Source: CAD feature listing. Evaluate the final solid. Frame: model axes, mm. A direction names the side the tool comes from. Give positions to 0.01 mm unless a question says otherwise; leave off trailing zeros. Order: outer loops, then holes, each group sorted by start corner. A loop starts at its lowest first (then second) coordinate and runs counter-clockwise, first axis right, second up. Notation, with made-up numbers: (-4.75, 19) -> (43.25, 19) arc R19 cw to (43.25, 38) -> close; hole circle Ø6 at (26, 9.5). An arc over 180 degrees is marked (long way). Use CSV: the item, a comma, the result in double quotes.
```python
from build123d import *

# Parameters (mm, degrees)
SKETCH1_R                = 7.6
BOSS_EXTRUDE1_DEPTH      = 2
M4_CLEARANCE_HOLE1_D     = 4.3
M4_CLEARANCE_HOLE1_DEPTH = 8
M4_CLEARANCE_HOLE1_TIP   = 1.291850331


with BuildPart() as part:
    # Sketch1 → Boss-Extrude1 (new body)
    with BuildSketch(Plane(origin=(0, 0, 0), x_dir=(1, 0, 0), z_dir=(0, 1, 0))):
        with BuildLine():
            ThreePointArc((-4.926264158, -18.505524079), (0, -22.65), (4.926264158, -18.505524079))
            ThreePointArc((4.926264158, -18.505524079), (13.54109486, -13.54109486), (18.505524079, -4.926264158))
            ThreePointArc((18.505524079, -4.926264158), (22.65, 0), (18.505524079, 4.926264158))
            ThreePointArc((18.505524079, 4.926264158), (13.54109486, 13.54109486), (4.926264158, 18.505524079))
            ThreePointArc((4.926264158, 18.505524079), (0, 22.65), (-4.926264158, 18.505524079))
            ThreePointArc((-4.926264158, 18.505524079), (-13.54109486, 13.54109486), (-18.505524079, 4.926264158))
            ThreePointArc((-18.505524079, 4.926264158), (-22.65, 0), (-18.505524079, -4.926264158))
            ThreePointArc((-18.505524079, -4.926264158), (-13.54109486, -13.54109486), (-4.926264158, -18.505524079))
        make_face()
        with BuildLine():
            ThreePointArc((-4.516771305, -15.505524079), (-11.419774516, -11.419774516), (-15.505524079, -4.516771305))
            ThreePointArc((-15.505524079, -4.516771305), (-14.21735127, -3.635508588), (-13.26365756, -2.4))
            Line((-13.26365756, -2.4), (-10.73498952, -2.4))
            ThreePointArc((-10.73498952, -2.4), (-7.778174593, -7.778174593), (-2.4, -10.73498952))
            Line((-2.4, -10.73498952), (-2.4, -13.26365756))
            ThreePointArc((-2.4, -13.26365756), (-3.635508588, -14.21735127), (-4.516771305, -15.505524079))
        make_face(mode=Mode.SUBTRACT)
        with BuildLine():
            ThreePointArc((4.516771305, -15.505524079), (3.635508588, -14.21735127), (2.4, -13.26365756))
            Line((2.4, -13.26365756), (2.4, -10.73498952))
            ThreePointArc((2.4, -10.73498952), (7.778174593, -7.778174593), (10.73498952, -2.4))
            Line((10.73498952, -2.4), (13.26365756, -2.4))
            ThreePointArc((13.26365756, -2.4), (14.21735127, -3.635508588), (15.505524079, -4.516771305))
            ThreePointArc((15.505524079, -4.516771305), (11.419774516, -11.419774516), (4.516771305, -15.505524079))
        make_face(mode=Mode.SUBTRACT)
        with BuildLine():
            Line((-10.73498952, 2.4), (-13.26365756, 2.4))
            ThreePointArc((-13.26365756, 2.4), (-14.21735127, 3.635508588), (-15.505524079, 4.516771305))
            ThreePointArc((-15.505524079, 4.516771305), (-11.419774516, 11.419774516), (-4.516771305, 15.505524079))
            ThreePointArc((-4.516771305, 15.505524079), (-3.635508588, 14.21735127), (-2.4, 13.26365756))
            Line((-2.4, 13.26365756), (-2.4, 10.73498952))
            ThreePointArc((-2.4, 10.73498952), (-7.778174593, 7.778174593), (-10.73498952, 2.4))
        make_face(mode=Mode.SUBTRACT)
        with Locations(Location((0, 0, 0), (0, 0, 270))):
            Circle(SKETCH1_R, mode=Mode.SUBTRACT)
        with BuildLine():
            Line((2.4, 10.73498952), (2.4, 13.26365756))
            ThreePointArc((2.4, 13.26365756), (3.635508588, 14.21735127), (4.516771305, 15.505524079))
            ThreePointArc((4.516771305, 15.505524079), (11.419774516, 11.419774516), (15.505524079, 4.516771305))
            ThreePointArc((15.505524079, 4.516771305), (14.21735127, 3.635508588), (13.26365756, 2.4))
            Line((13.26365756, 2.4), (10.73498952, 2.4))
            ThreePointArc((10.73498952, 2.4), (7.778174593, 7.778174593), (2.4, 10.73498952))
        make_face(mode=Mode.SUBTRACT)
    extrude(amount=BOSS_EXTRUDE1_DEPTH)

    # M4 Clearance Hole1
    with Locations(Plane(origin=(0, 0, 0), x_dir=(-1, 0, 0), z_dir=(0, -1, 0))):
        with Locations((-17.65, 0), (0, 17.65), (17.65, 0), (0, -17.65)):
            Hole(M4_CLEARANCE_HOLE1_D / 2, depth=M4_CLEARANCE_HOLE1_DEPTH)
            with Locations((0, 0, -(M4_CLEARANCE_HOLE1_DEPTH + M4_CLEARANCE_HOLE1_TIP / 2))):  # 118° drill point
                Cone(0, M4_CLEARANCE_HOLE1_D / 2, M4_CLEARANCE_HOLE1_TIP, mode=Mode.SUBTRACT)


solid = part.part
```
1. Mould query, pull axis X, two halves, no side actions, for faces 3 (the cylindrical face through (-13.64, 0.99, 13.44)), 4 (the flat face through (-12, 1, 2.4)), 5 (the cylindrical face through (22.65, 0.99, 0.1)), 6 (the cylindrical face through (7.716, 0.986, 7.84)). Classes: released by +X, released by -X, zero draft, split by the parting line, or undercut.
Answer below:
face 3,"released by -X"
face 4,"undercut"
face 5,"released by +X"
face 6,"undercut"
2. Section query A-A on z = 0. Return loops of the section in (x, y).
Answer below:
outline,"(-22.65, 0) -> (-19.8, 0) -> (-19.8, 2) -> (-22.65, 2) -> close; (-15.5, 0) -> (-7.6, 0) -> (-7.6, 2) -> (-15.5, 2) -> close; (7.6, 0) -> (15.5, 0) -> (15.5, 2) -> (7.6, 2) -> close; (19.8, 0) -> (22.65, 0) -> (22.65, 2) -> (19.8, 2) -> close"
3. Ray query, line 1 along X through (y, z) = (1.75, 9); line 2 along Z through (x, y) = (-6, 0.85); line 3 along Z through (x, y) = (15, 1.5). Return the intervals inside material, ascending.
Answer below:
line 1,"x = -16.9 to -13.41, -6.32 to 6.32, 13.41 to 16.9"
line 2,"z = -18.19 to -14.99, -9.22 to -4.66, 4.66 to 9.22, 14.99 to 18.19"
line 3,"z = -11.9 to -5.99, -4.24 to 4.24, 5.99 to 11.9"
4. Section query B-B on x = 0. Return loops of the section in (y, z).
Answer below:
outline,"(0, -22.65) -> (2, -22.65) -> (2, -19.8) -> (0, -19.8) -> close; (0, -15.5) -> (2, -15.5) -> (2, -7.6) -> (0, -7.6) -> close; (0, 7.6) -> (2, 7.6) -> (2, 15.5) -> (0, 15.5) -> close; (0, 19.8) -> (2, 19.8) -> (2, 22.65) -> (0, 22.65) -> close"
5. Pin query (flat end, axial travel): P1, Ø5, axis at x = -17.65, z = 0, coming from the -Y side; P2, Ø0.6, axis at y = 1.5, z = -12.5, coming from the +X side; P3, Ø1, axis at y = 1, z = -12.5, coming from the -X side; P4, Ø0.6, axis at y = 1, z = 12, coming from the -X side. Return the tip coordinate at first contact, or that it passes through.
Answer below:
P1,"stops at y = 0"
P2,"stops at x = 14.76"
P3,"stops at x = -14.92"
P4,"stops at x = -15.16"
6. Section query C-C on x = -14. Return loops of the section in (y, z).
Answer below:
outline,"(0, -13.07) -> (2, -13.07) -> (2, -8.05) -> (0, -8.05) -> close; (0, -3.42) -> (2, -3.42) -> (2, 3.42) -> (0, 3.42) -> close; (0, 8.05) -> (2, 8.05) -> (2, 13.07) -> (0, 13.07) -> close"
7. Section query D-D on x = 17. Return loops of the section in (y, z).
Answer below:
outline,"(0, -8.82) -> (2, -8.82) -> (2, -2.05) -> (0, -2.05) -> close; (0, 2.05) -> (2, 2.05) -> (2, 8.82) -> (0, 8.82) -> close"
8. Access query for faces 1 (the cylindrical face through (13.64, 0.99, -13.44)), 2 (the cylindrical face through (11.34, 0.99, -11.5)). Directions: +Z, -Z, +X, -X, +Y, -Y. A direction counts if a zero-diameter tool reaches every point of the face in a straight line with its end or side. Return the directions, or none.
Answer below:
face 1,"-Z, +X, +Y, -Y"
face 2,"+Y, -Y"
